from build123d import *

# Parameters (mm, degrees)
F0_W     = 39
F0_H     = 16
F1_DEPTH = 2
F2_W     = 7
F2_H     = 13
F3_DEPTH = 6
F4_D     = 3
F5_D     = 4
F5_DEPTH = 2.001


with BuildPart() as f1:
    # F0 (on Top) → F1 (new body)
    with BuildSketch(Plane.XY):
        Rectangle(F0_W, F0_H)
    extrude(amount=F1_DEPTH)

    # F2 (on face) → F3 (join)
    with BuildSketch(Plane.XY.offset(2)):
        Polygon((-13.5, -2), (-13.5, -8), (-3, -8), (-0.5, -8), (-0.5, -2), align=None)
        with Locations((12, 0)):
            Rectangle(F2_W, F2_H)
        Polygon((-0.5, -8), (-3, -8), (-15.2969384567, -10.5101020514), (-15.1969384567, -11), align=None)
    extrude(amount=F3_DEPTH)

    # F4 (through all)
    with Locations(Plane.XY.offset(2)):
        with Locations((-16.5, -5), (2.5, -5)):
            Hole(F4_D / 2)

    # F5 (through all, one way)
    with BuildSketch(Plane.XY.offset(2)):
        with Locations((17, 5.5), (17, -5.5)):
            Circle(F5_D / 2)
    extrude(amount=-F5_DEPTH, mode=Mode.SUBTRACT)


solid = f1.part
Here's how the part is built. I have some questions about the finished solid (model axes, mm). A direction names the side the tool comes from. Round coordinates to 2 decimals unless told otherwise and drop trailing zeros. Order: outer loops, then holes, each group sorted by start corner. A loop starts at its lowest first (then second) coordinate and runs counter-clockwise, first axis right, second up. Notation, with made-up numbers: (45, -28) -> (75, -28) arc R13 cw to (75, -20) -> close; hole circle Ø5 at (-6, 78). An arc over 180 degrees is marked (long way). Use CSV: the item, a comma, the result in double quotes.
1. I want a section at C-C on y = -5.5. List the corners of the cut face in (x, z) for me, and give its area (3 significant figures).
Recorded:
outline,"(-19.5, 0) -> (-17.91, 0) -> (-17.91, 2) -> (-19.5, 2) -> close; (-15.09, 0) -> (1.09, 0) -> (1.09, 2) -> (-0.5, 2) -> (-0.5, 8) -> (-13.5, 8) -> (-13.5, 2) -> (-15.09, 2) -> close; (3.91, 0) -> (15, 0) -> (15, 2) -> (15.5, 2) -> (15.5, 8) -> (8.5, 8) -> (8.5, 2) -> (3.91, 2) -> close; (19, 0) -> (19.5, 0) -> (19.5, 2) -> (19, 2) -> close"
area,"179 mm2"
2. I want a section at A-A on x = 2.5. List the corners of the cut face in (y, z) for me, and give its area (3 significant figures).
Recorded:
outline,"(-8, 0) -> (-6.5, 0) -> (-6.5, 2) -> (-8, 2) -> close; (-3.5, 0) -> (8, 0) -> (8, 2) -> (-3.5, 2) -> close"
area,"26.0 mm2"
3. I want a section at B-B on z = 6.25. List the corners of the cut face in (x, y) for me.
Recorded:
outline,"(-15.3, -10.51) -> (-15.2, -11) -> (-0.5, -8) -> (-0.5, -2) -> (-13.5, -2) -> (-13.5, -8) -> (-3, -8) -> close; (8.5, -6.5) -> (15.5, -6.5) -> (15.5, 6.5) -> (8.5, 6.5) -> close"
4. I'm going to push flat-ended pins straight in: P1, Ø1.8, axis at x = -16.5, y = -5, coming from the +Z side; P2, Ø4, axis at x = -9.5, z = 1.5, coming from the -Y side; P3, Ø3, axis at x = 12.5, z = 4, coming from the +Y side; P4, Ø4, axis at x = -1, z = 4, coming from the -Y side. Where does each tip first touch, or does it pass through?
Recorded:
P1,"passes through"
P2,"stops at y = -10.23"
P3,"stops at y = 6.5"
P4,"stops at y = -8.51"
5. I want a section at D-D on x = 9. List the corners of the cut face in (y, z) for me.
Recorded:
outline,"(-8, 0) -> (8, 0) -> (8, 2) -> (6.5, 2) -> (6.5, 8) -> (-6.5, 8) -> (-6.5, 2) -> (-8, 2) -> close"
6. Which directions (+Z, -Z, +X, -X, +Y, -Y) give clear straight access to the entire face, cutting with the end or side of a thin tool? Please do faces 1 (the face through (12, -6.5, 5)), 2 (the face through (8.5, 0, 5)), 3 (the face through (15.526, 6.852, 1.014)), 4 (the face through (12, 6.5, 5)), 5 (the face through (15.5, 0, 5)).
Recorded:
face 1,"+Z, +X, -Y"
face 2,"+Z, +Y, -Y"
face 3,"-Z"
face 4,"+Z, +X, -X, +Y"
face 5,"+Z, +X, +Y, -Y"
7. I need wall thicknesses on line 1 along Y through (x, z) = (17, 1); line 2 along X through (y, z) = (5.5, 0.7); line 3 along Y through (x, z) = (-16.5, 1.1). Which ranges of each line are inside material? Lowest first, please.
Recorded:
line 1,"y = -8 to -7.5, -3.5 to 3.5, 7.5 to 8"
line 2,"x = -19.5 to 15, 19 to 19.5"
line 3,"y = -8 to -6.5, -3.5 to 8"
